```python
from build123d import *

# Parameters (mm, degrees)
CROQUIS1_R              = 17.5
CROQUIS1_R_2            = 6.35
SALIENTE_EXTRUIR1_DEPTH = 11
REDONDEO1_R             = 2
SALIENTE_EXTRUIR2_REACH = 29.083
CROQUIS2_W              = 0.263095083
CROQUIS2_H              = 1.425025485


with BuildPart() as part:
    # Croquis1 → Saliente-Extruir1 (new body)
    with BuildSketch(Plane.XY):
        Circle(CROQUIS1_R)
        Circle(CROQUIS1_R_2, mode=Mode.SUBTRACT)
    extrude(amount=SALIENTE_EXTRUIR1_DEPTH)

    # Redondeo1
    redondeo1_edges = [part.edges().sort_by_distance(p)[0] for p in [
        (-17.5, 0, 0),
        (-17.5, 0, 11),
    ]]
    fillet(redondeo1_edges, radius=REDONDEO1_R)

    # Saliente-Extruir2: up to this face of the body (flat: up to its plane)
    saliente_extruir2_end = Plane(part.part.faces().sort_by_distance((-15.061593796, 0, 0))[0])
    # Croquis2 → Saliente-Extruir2 (add, up to the picked face)
    with BuildSketch(Plane.XY.offset(11), mode=Mode.PRIVATE) as saliente_extruir2_sk1:
        with Locations((-17.368452459, -0.712512743)):
            Rectangle(CROQUIS2_W, CROQUIS2_H)
    saliente_extruir2_tool1 = split(extrude(saliente_extruir2_sk1.sketch, amount=-SALIENTE_EXTRUIR2_REACH, mode=Mode.PRIVATE), bisect_by=saliente_extruir2_end, keep=Keep.BOTH, mode=Mode.PRIVATE)
    add(saliente_extruir2_tool1.solids().sort_by(Axis((-17.368452, -0.712513, 11), (0, 0, -1)))[0])


solid = part.part
```
Part model, mm, in its own coordinate system. Round coordinates to 2 decimals unless told otherwise and drop trailing zeros. Write each loop counter-clockwise with the first axis right and the second up, starting at its lowest first coordinate (ties: lowest second). Pieces come first, ordered by that corner, then holes. Notation, with made-up numbers: (26.5, 23) -> (57.5, 23) arc R28 ccw to (57.5, 60) -> close; hole circle Ø3 at (-25.75, 56). An arc over 180 degrees is marked (long way). Return JSON: item names as keys, results as strings. Group by question number.
Q1. Saw through at A-A on x = 0. Write the cut outline in (y, z), plus the area to 3 significant figures.
Q2. Probe L1, parallel to Y at x = 0, z = 4.5; L2, parallel to Z at x = 14.5, y = 6; L3, parallel to X at y = -4, z = 2.25. List the from-to ranges inside material, lowest first. Write a range as [from, to].
Q3. Mould opens along X. For faces 1 (the flat face through (-17.5, -1, 6)), 2 (the flat face through (-17.237, -0.7, 10.4)), 3 (the flat face through (0, -7, 11)) say: pulls with the +X half, pulls with the -X half, needs draft (parallel to the pull), parting line crosses it, or undercut.
Q4. Saw through at B-B on z = 7.75. Write the cut outline in (x, y), plus the area to 3 significant figures.
Q5. Pin check, flat tips, straight feed: pin 1 (4 mm diameter, centred on x = 10, z = 6.5, fed in from +Y); pin 2 (4 mm diameter, centred on y = 4, z = 8, fed in from -X); pin 3 (6 mm diameter, centred on x = -5.5, z = 5, fed in from -Y). Stop position of each tip, or through.
Answer:
{
 "1": {"outline": "(-17.5, 2) arc R2 ccw to (-15.5, 0) -> (-6.35, 0) -> (-6.35, 11) -> (-15.5, 11) arc R2 ccw to (-17.5, 9) -> close; (6.35, 0) -> (15.5, 0) arc R2 ccw to (17.5, 2) -> (17.5, 9) arc R2 ccw to (15.5, 11) -> (6.35, 11) -> close", "area": "242 mm2"},
 "2": {"L1": "[-17.5, -6.35], [6.35, 17.5]", "L2": "[0.01, 10.99]", "L3": "[-17.04, -4.93], [4.93, 17.04]"},
 "3": {"face 1": "pulls with the -X half", "face 2": "undercut", "face 3": "needs draft"},
 "4": {"outline": "(-17.5, -1.43) -> (-17.44, -1.43) arc R17.5 ccw (long way) to (-17.5, 0) -> close; hole circle Ø12.7 at (0, 0)", "area": "835 mm2"},
 "5": {"pin 1": "y = 15.56", "pin 2": "x = -17.39", "pin 3": "y = -17.32"}
}
